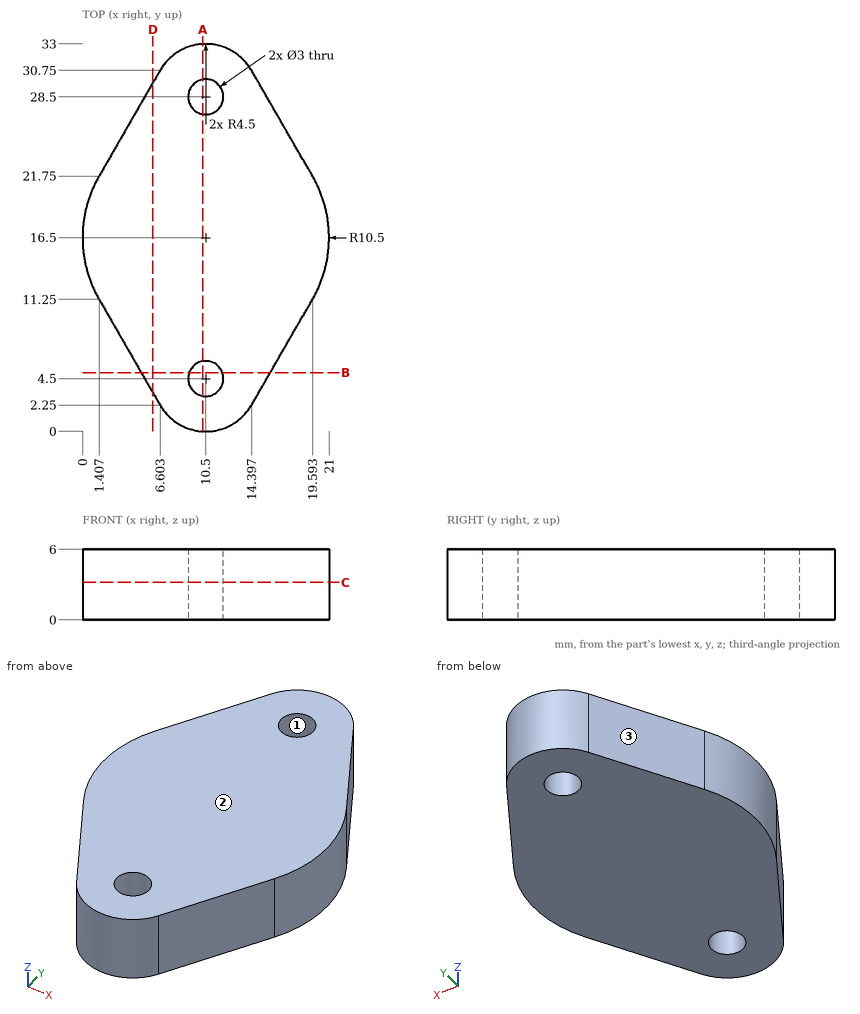
Source: three-view drawing plus pictorial views. Frame: mm from the lowest corner of the part. Coordinates: 2 decimals unless noted, no trailing zeros. Order: outer loops, then holes, each group sorted by start corner. A loop starts at its lowest first (then second) coordinate and runs counter-clockwise, first axis right, second up.
1) Section C-C (z = 3.2). Return loops of the section in (x, y).
Result sheet:
outline: (1.41, 11.25) - (6.6, 2.25) arc R4.5 ccw to (14.4, 2.25) - (19.59, 11.25) arc R10.5 ccw to (19.59, 21.75) - (14.4, 30.75) arc R4.5 ccw to (6.6, 30.75) - (1.41, 21.75) arc R10.5 ccw to start; hole circle Ø3 at (10.5, 4.5); hole circle Ø3 at (10.5, 28.5)
2) Section D-D (x = 6). Return loops of the section in (y, z).
Result sheet:
outline: (3.29, 0) - (29.71, 0) - (29.71, 6) - (3.29, 6) - close
3) Section B-B (y = 5). Return loops of the section in (x, z) (1 decimal).
Result sheet:
outline: (5, 0) - (9.1, 0) - (9.1, 6) - (5, 6) - close; (11.9, 0) - (16, 0) - (16, 6) - (11.9, 6) - close
4) Draft query along Y for the marked faces 1, 2 and 3. Return one class per face: released by +Y, released by -Y, zero draft, split by the parting line, or undercut.
Result sheet:
face 1: undercut
face 2: zero draft
face 3: released by +Y
5) First-contact query: P1, Ø3, axis at y = 5.5, z = 5.5, coming from the -X side; P2, Ø1, axis at y = 20.5, z = 4, coming from the +X side; P3, Ø3, axis at x = 4, z = 5.5, coming from the -Y side. Flat tips, straight axial feed; report the tip coordinate or a pass-through.
Result sheet:
P1: stops at x = 3.86
P2: stops at x = 20.4
P3: stops at y = 4.16
6) Ray query, probe 1 along Y at (x, z) = (9.5, 3.85); probe 2 along Y at (x, z) = (8, 4.3); probe 3 along Y at (x, z) = (19.25, 4.1) (1 decimal). Return the intervals inside material, ascending.
Result sheet:
probe 1: y = 0.11 to 3.38, 5.62 to 27.38, 29.62 to 32.89
probe 2: y = 0.76 to 32.24
probe 3: y = 10.7 to 22.3
7) Section A-A (x = 10.25). Return loops of the section in (y, z), then the cut area to 3 significant figures.
Result sheet:
outline: (0.01, 0) - (3.02, 0) - (3.02, 6) - (0.01, 6) - close; (5.98, 0) - (27.02, 0) - (27.02, 6) - (5.98, 6) - close; (29.98, 0) - (32.99, 0) - (32.99, 6) - (29.98, 6) - close
area: 162 mm2
